Part print with two shaded views. Sizes in mm from the minimum x, y, z corner. A direction names the side the tool comes from. Round coordinates to 2 decimals unless told otherwise and drop trailing zeros. Order: outer loops, then holes, each group sorted by start corner. A loop starts at its lowest first (then second) coordinate and runs counter-clockwise, first axis right, second up. Notation, with made-up numbers: M -32.5,31 L 24.5,31 A8 ccw 24.5,45 Z; hole C -0.5,-35 d4. An arc over 180 degrees is marked long. Return JSON: item names as keys, results as strings. Group by question number.
Item 1: Probe line 1 along Z through (x, y) = (19.75, 15); line 2 along Y through (x, z) = (15, 7.5); line 3 along X through (y, z) = (12, 0.75) (1 decimal). List the from-to ranges inside material, lowest first.
Item 2: Slice it at D-D on x = 9.5. Write the cut outline in (y, z), then the cut area to 3 significant figures.
Item 3: Slice it at B-B on y = 8.5. Write the cut outline in (x, z), then the cut area to 3 significant figures.
Item 4: Which spindle directions (+Z, -Z, +X, -X, +Y, -Y) get a long thin tool onto all of the face, cutting with end or side? Do the marked faces 1 and 2. Say none if no direction does.
Item 5: Slice it at C-C on x = 12.5. Write the cut outline in (y, z), then the cut area to 3 significant figures.
Item 6: Pull direction Z, two halves, no side cores. Call the marked faces 3, 4 and 5: pulls with the +Z half, pulls with the -Z half, needs draft (parallel to the pull), parting line crosses it, or undercut.
Item 7: Slice it at A-A on y = 14. Write the cut outline in (x, z).
Item 8: Pin check, flat tips, straight feed: pin 1 Ø1.5 at (y, z) = (9, 2.5) entering from -X; pin 2 Ø8 at (y, z) = (17.5, 7) entering from +X. Stop position of each tip, or through.
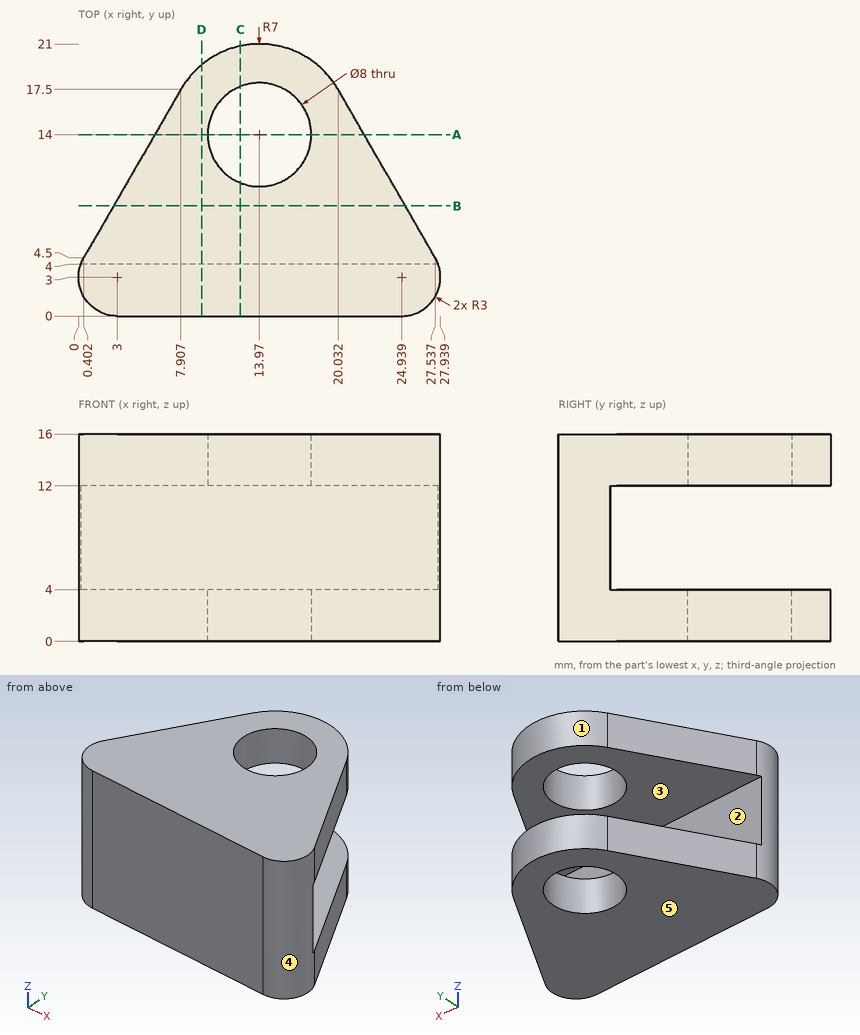
Output values:
{
 "1": {"line 1": "0 to 4, 12 to 16", "line 2": "0 to 4", "line 3": "4.7 to 10.5, 17.4 to 23.2"},
 "2": {"outline": "M 0,0 L 19.39,0 L 19.39,4 L 4,4 L 4,12 L 19.39,12 L 19.39,16 L 0,16 Z", "area": "187 mm²"},
 "3": {"outline": "M 2.71,0 L 25.23,0 L 25.23,4 L 2.71,4 Z; M 2.71,12 L 25.23,12 L 25.23,16 L 2.71,16 Z", "area": "180 mm²"},
 "4": {"face 1": "+Z, -Z, +Y", "face 2": "+X, -X, +Y"},
 "5": {"outline": "M 0,0 L 10.28,0 L 10.28,4 L 4,4 L 4,12 L 10.28,12 L 10.28,16 L 0,16 Z; M 17.72,0 L 20.84,0 L 20.84,4 L 17.72,4 Z; M 17.72,12 L 20.84,12 L 20.84,16 L 17.72,16 Z", "area": "139 mm²"},
 "6": {"face 3": "undercut", "face 4": "needs draft", "face 5": "pulls with the -Z half"},
 "7": {"outline": "M 5.89,0 L 9.97,0 L 9.97,4 L 5.89,4 Z; M 5.89,12 L 9.97,12 L 9.97,16 L 5.89,16 Z; M 17.97,0 L 22.05,0 L 22.05,4 L 17.97,4 Z; M 17.97,12 L 22.05,12 L 22.05,16 L 17.97,16 Z"},
 "8": {"pin 1": "x = 2.57", "pin 2": "x = 21.56"}
}
